Check sheet for the modelled part. Datum: model origin and axes. Units: mm. Give positions to 0.01 mm unless a question says otherwise; leave off trailing zeros. Loops run counter-clockwise (first coordinate to the right, second up) from the corner with the lowest first, then second, coordinate; pieces in that order, holes last. Notation, with made-up numbers: M -33,68.25 L 23,68.25 A32 ccw 23,94.25 Z; hole C 14,16.25 d5. An arc over 180 degrees is marked long. One line per question, with ' | ' between items. Start each with the question number.
from build123d import *

# Parameters (mm, degrees)
F0_W          = 2.5
F0_H          = 2.5
F0_W_2        = 20
F0_H_2        = 60
F0_W_3        = 40
F1_DEPTH      = 15
F2_W          = 20
F2_H          = 10
F2_W_2        = 40
F3_DEPTH      = 70
F4_W          = 10
F4_H          = 60
F5_DEPTH      = 25
F5_DEPTH_BACK = 25


with BuildPart() as f1:
    # F0 (on Front) → F1 (new body)
    with BuildSketch(Plane.XZ):
        with Locations((-11.25, 63.75)):
            Rectangle(F0_W, F0_H)
        with Locations((0, 63.75)):
            Rectangle(F0_W_2, F0_H)
        with Locations((11.25, 63.75)):
            Rectangle(F0_W, F0_H)
        with Locations((-11.25, 32.5)):
            Rectangle(F0_W, F0_H_2)
        with Locations((11.25, 32.5)):
            Rectangle(F0_W, F0_H_2)
        with Locations((0, 1.25)):
            Rectangle(F0_W_2, F0_H)
        with Locations((-32.5, 1.25)):
            Rectangle(F0_W_3, F0_H)
        with Locations((32.5, 1.25)):
            Rectangle(F0_W_3, F0_H)
        with Locations((11.25, 1.25)):
            Rectangle(F0_W, F0_H)
        with Locations((53.75, 1.25)):
            Rectangle(F0_W, F0_H)
        with Locations((-11.25, 1.25)):
            Rectangle(F0_W, F0_H)
        with Locations((-53.75, 1.25)):
            Rectangle(F0_W, F0_H)
    extrude(amount=F1_DEPTH)

    # F2 (on Top) → F3 (cut)
    with BuildSketch(Plane.XY):
        with Locations((0, -7.5)):
            Rectangle(F2_W, F2_H)
        with Locations((32.5, -7.5)):
            Rectangle(F2_W_2, F2_H)
        with Locations((-32.5, -7.5)):
            Rectangle(F2_W_2, F2_H)
    extrude(amount=F3_DEPTH, mode=Mode.SUBTRACT)

    # F4 (on Right) → F5 (cut, two sides)
    with BuildSketch(Plane.YZ) as f5_sk:
        with Locations((-7.5, 32.5)):
            Rectangle(F4_W, F4_H)
    extrude(amount=-F5_DEPTH, mode=Mode.SUBTRACT)
    extrude(f5_sk.sketch, amount=F5_DEPTH_BACK, mode=Mode.SUBTRACT)


solid = f1.part
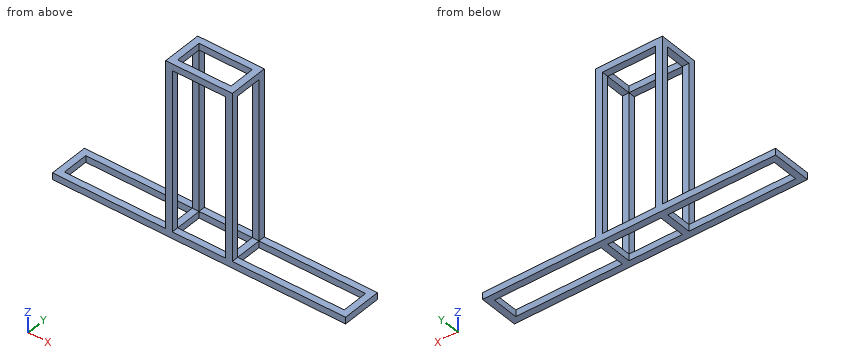
Q1. Cross-section at D-D (z = 10.5). Record the cut outline in (x, y).
Q2. Cross-section at B-B (x = -1). Record the cut outline in (y, z).
Q3. Depth check by flat-ended pin: P1, Ø4, axis at y = -11, z = 13.5, coming from the -X side; P2, Ø0.8, axis at y = -8, z = 64, coming from the +X side. Enter the tip coordinate at first touch or a pass-through.
Q4. Cross-section at A-A (y = -4.75). Record the cut outline in (x, z).
Q5. Cross-section at C-C (x = -22). Record the cut outline in (y, z), and give its area (3 significant figures).
Q6. Material ranges on probe 1 along X at (y, z) = (-0.25, 30); probe 2 along Z at (x, y) = (-5, -14); probe 3 along Z at (x, y) = (-48, -2), recorded low to high. Write a range as from..to.
Solved:
1) outline: M -12.5,-15 L -10,-15 L -10,-12.5 L -12.5,-12.5 Z; M -12.5,-2.5 L -10,-2.5 L -10,0 L -12.5,0 Z; M 10,-15 L 12.5,-15 L 12.5,-12.5 L 10,-12.5 Z; M 10,-2.5 L 12.5,-2.5 L 12.5,0 L 10,0 Z
2) outline: M -15,0 L -12.5,0 L -12.5,2.5 L -15,2.5 Z; M -15,62.5 L -12.5,62.5 L -12.5,65 L -15,65 Z; M -2.5,0 L 0,0 L 0,2.5 L -2.5,2.5 Z; M -2.5,62.5 L 0,62.5 L 0,65 L -2.5,65 Z
3) P1: stops at x = -12.5 | P2: stops at x = 12.5
4) outline: M -55,0 L -52.5,0 L -52.5,2.5 L -55,2.5 Z; M -12.5,0 L -10,0 L -10,2.5 L -12.5,2.5 Z; M -12.5,62.5 L -10,62.5 L -10,65 L -12.5,65 Z; M 10,0 L 12.5,0 L 12.5,2.5 L 10,2.5 Z; M 10,62.5 L 12.5,62.5 L 12.5,65 L 10,65 Z; M 52.5,0 L 55,0 L 55,2.5 L 52.5,2.5 Z
5) outline: M -15,0 L -12.5,0 L -12.5,2.5 L -15,2.5 Z; M -2.5,0 L 0,0 L 0,2.5 L -2.5,2.5 Z | area: 12.5 mm²
6) probe 1: x = -12.5..-10, 10..12.5 | probe 2: z = 0..2.5, 62.5..65 | probe 3: z = 0..2.5
